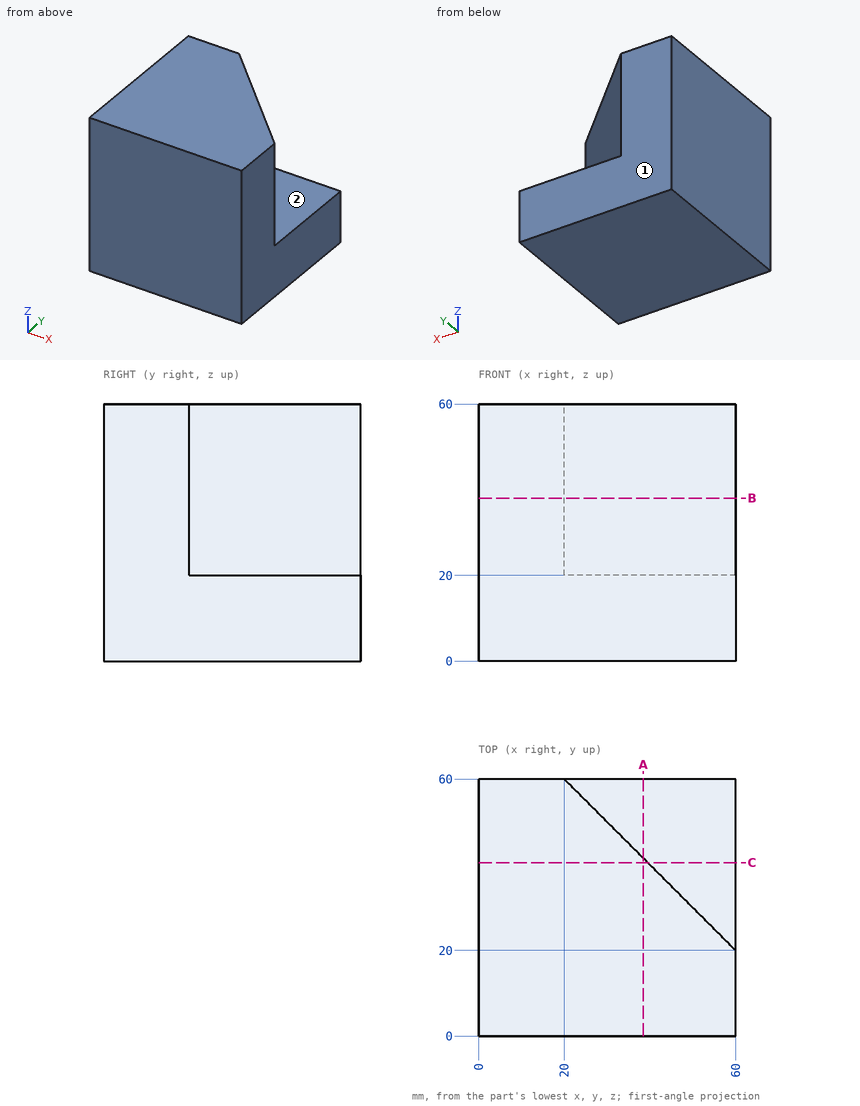
The figure shows three views and two pictorial views of one solid part (mm, origin at its lowest corner). Answer the questions. A direction names the side the tool comes from. Round coordinates to 2 decimals unless told otherwise and drop trailing zeros. Write each loop counter-clockwise with the first axis right and the second up, starting at its lowest first coordinate (ties: lowest second). Pieces come first, ordered by that corner, then holes. Notation, with made-up numbers: M 76,-20.75 L 126,-20.75 A12 cw 126,-6.75 Z; hole C 50,60 d7. An arc over 180 degrees is marked long. Use a Markdown table: item, result.
1) The part is cut by section C-C on y = 40.5. Give the vertices of the cut face in (x, z).
Taken from the geometry:
| item | result |
|---|---|
| outline | M 0,0 L 60,0 L 60,20 L 39.5,20 L 39.5,60 L 0,60 Z |
2) Which of the six approach directions +Z, -Z, +X, -X, +Y, -Y give full straight-line access (tool end or side, diameter ignored) to the marked faces 1 and 2?
Taken from the geometry:
| item | result |
|---|---|
| face 1 | +Z, -Z, +X, -X, +Y |
| face 2 | +Z, +X, +Y |
3) Consider line 1 (Z direction, x = 51, y = 44); line 2 (X direction, y = 23, z = 38.5); line 3 (X direction, y = 44, z = 23). Determine where each line is inside the solid, lowest interval first. Write a range as [from, to].
Taken from the geometry:
| item | result |
|---|---|
| line 1 | z = [0, 20] |
| line 2 | x = [0, 57] |
| line 3 | x = [0, 36] |
4) The part is cut by section A-A on x = 38.5. Give the vertices of the cut face in (y, z).
Taken from the geometry:
| item | result |
|---|---|
| outline | M 0,0 L 60,0 L 60,20 L 41.5,20 L 41.5,60 L 0,60 Z |
5) The part is cut by section B-B on z = 38. Give the vertices of the cut face in (x, y), plus the area to 3 significant figures.
Taken from the geometry:
| item | result |
|---|---|
| outline | M 0,0 L 60,0 L 60,20 L 20,60 L 0,60 Z |
| area | 2,800 mm2 |
6) Flat-ended cylindrical pins translate along their axes: pin 1 (3 mm diameter, centred on x = 38, y = 49, fed in from +Z); pin 2 (4 mm diameter, centred on x = 45, z = 40.5, fed in from +Y); pin 3 (1.5 mm diameter, centred on y = 25.5, z = 30, fed in from +X). Find the tip coordinate at first contact, or state that the pin passes through.
Taken from the geometry:
| item | result |
|---|---|
| pin 1 | stops at z = 20 |
| pin 2 | stops at y = 37 |
| pin 3 | stops at x = 55.25 |
